from build123d import *

# Parameters (mm, degrees)
BOSS_EXTRUDE1_DEPTH      = 187
SKETCH3_R                = 1.5
CUT_EXTRUDE2_DEPTH       = 188
CUT_EXTRUDE1_DEPTH       = 3
BOSS_EXTRUDE2_DEPTH      = 2
BOSS_EXTRUDE2_DEPTH_BACK = 189


with BuildPart() as part:
    # Sketch1 → Boss-Extrude1 (new body)
    with BuildSketch(Plane.XY):
        with BuildLine():
            Line((0, 0), (0, 5))
            Line((0, 5), (5, 5))
            Line((5, 5), (10, 0))
            Line((10, 0), (10, -5))
            Line((10, -5), (5, -5))
            ThreePointArc((5, -5), (1.464466094, -3.535533906), (0, 0))
        make_face()
    extrude(amount=BOSS_EXTRUDE1_DEPTH)

    # Sketch3 → Cut-Extrude2 (cut, through all)
    with BuildSketch(Plane.XY.offset(187)):
        with Locations((5, 0)):
            Circle(SKETCH3_R)
    extrude(amount=-CUT_EXTRUDE2_DEPTH, mode=Mode.SUBTRACT)

    # Sketch2 → Cut-Extrude1 (cut)
    with BuildSketch(Plane.ZY):
        Polygon((178, 0.5), (9, 0.5), (0, 4.5), (0, 5), (187, 5), (187, 4.5), align=None)
    cut_extrude1 = extrude(amount=-CUT_EXTRUDE1_DEPTH, mode=Mode.SUBTRACT)

    # Mirror1: Cut-Extrude1 across plane
    add(cut_extrude1.mirror(Plane(origin=(2.5, -2.5, 0), x_dir=(0, 0, 1), z_dir=(-0.707106781, 0.707106781, 0))), mode=Mode.SUBTRACT)

    # Sketch4 → Boss-Extrude2 (add, two sides)
    with BuildSketch(Plane.XY.offset(187)) as boss_extrude2_sk:
        Polygon((5.201902961, 4.798097039), (9.798097039, 0.201902961), (8.560660172, -1.035533906), (3.964466094, 3.560660172), align=None)
    extrude(amount=BOSS_EXTRUDE2_DEPTH)
    extrude(boss_extrude2_sk.sketch, amount=-BOSS_EXTRUDE2_DEPTH_BACK)


solid = part.part
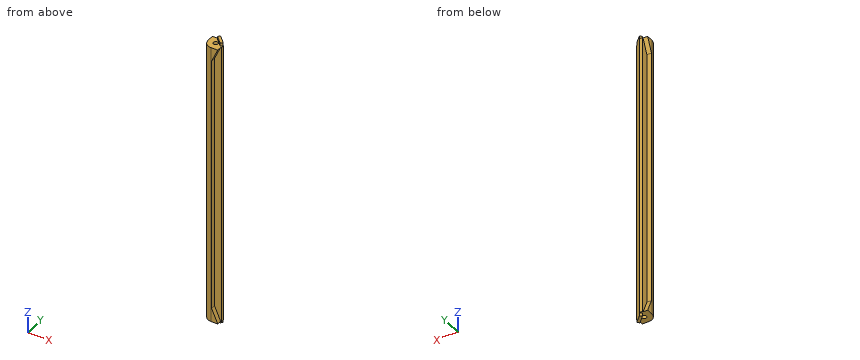
The model under review builds one solid part; all positions refer to its coordinate system, in mm. Round coordinates to 2 decimals unless told otherwise and drop trailing zeros. Loops run counter-clockwise (first coordinate to the right, second up) from the corner with the lowest first, then second, coordinate; pieces in that order, holes last. Notation, with made-up numbers: M 67.25,7 L 110.25,7 A24 ccw 110.25,20 Z; hole C 4.5,86 d4. An arc over 180 degrees is marked long. Answer as CSV lines item,"result". Start each with the question number.
Item 1: Consider section A-A (z = 132). Write out the cut boundary in (x, y).
Item 2: Insertion check: P1, Ø1.3, axis at y = 3, z = 87, coming from the -X side; P2, Ø2, axis at x = 3, z = 75, coming from the -Y side; P3, Ø6, axis at y = 3.5, z = 113, coming from the +X side. Each pin has a flat end and moves straight along its axis. Give the tip position at first contact, or say it passes through.
Item 3: Wall thickness on line 1 (Y direction, x = 5, z = 57); line 2 (Z direction, x = 2, y = -0.5); line 3 (X direction, y = 3.5, z = 19): over which ranges is each line inside the solid? List them lowest first. Write a range as [from, to].
Answer:
1,outline,"M 0,0 A5 ccw 5,-5 L 5.5,-5 L 5.5,-2 L 10,-2 L 10,0 L 5,5 L 3,5 L 3,0.5 L 0,0.5 Z; hole C 5,0 d3"
2,P1,"stops at x = 3"
2,P2,"stops at y = -4.9"
2,P3,"stops at x = 9.5"
3,line 1,"y = [-5, -1.5], [1.5, 5]"
3,line 2,"z = [0, 187]"
3,line 3,"x = [3, 6.5]"
